Read the model definition and answer for the solid it produces. Units are mm, in the model's axes. Face numbers are marked on the shaded views. A direction names the side the tool comes from. Give positions to 0.01 mm unless a question says otherwise; leave off trailing zeros. Write each loop counter-clockwise with the first axis right and the second up, starting at its lowest first coordinate (ties: lowest second). Pieces come first, ordered by that corner, then holes. Notation, with made-up numbers: M -8.5,-28.75 L 5.5,-28.75 A17 ccw 5.5,-11.75 Z; hole C 25.5,-8 d8. An arc over 180 degrees is marked long. Put each result on its own line as item: value.
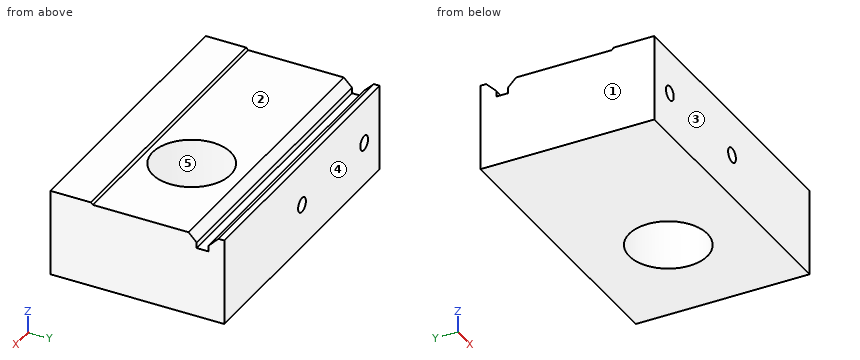
from build123d import *

# Parameters (mm, degrees)
SKETCH1_W                   = 100
SKETCH1_H                   = 60
BOSS_EXTRUDE1_DEPTH         = 30
CUT_EXTRUDE1_DEPTH          = 110
SKETCH_1_R                  = 2.5
CUT_EXTRUDE_1_DEPTH         = 10
PATTERN_LINEAR_1_COUNT      = 2
PATTERN_LINEAR_1_PITCH      = 40
PATTERN_LINEAR_1_COUNT_DIR2 = 2
PATTERN_LINEAR_1_PITCH_DIR2 = 50
SKETCH_2_R                  = 13.5
CUT_EXTRUDE_2_DEPTH         = 100


with BuildPart() as part:
    # Sketch1 → Boss-Extrude1 (new body)
    with BuildSketch(Plane.XY):
        with Locations((2.079207921, -0.485148515)):
            Rectangle(SKETCH1_W, SKETCH1_H)
    extrude(amount=BOSS_EXTRUDE1_DEPTH)

    # Sketch3 → Cut-Extrude1 (cut)
    with BuildSketch(Plane.ZY.offset(47.920792079)):
        Polygon((30, -30.485148515), (30, -16.485148515), (29.292893219, -15.778041734), (29.292893219, 17.150890454), (26.464466094, 19.979317579), (24.464466094, 19.979317579), (24.464466094, 23.979317579), (26.464466094, 23.979317579), (30, 27.514851485), (30, 29.514851485), (35.630972976, 28.601630178), (37.149112702, -26.247837132), align=None)
    extrude(amount=-CUT_EXTRUDE1_DEPTH, mode=Mode.SUBTRACT)

    # Эскиз1 → Вырез-Вытянуть1 (cut)
    with BuildSketch(Plane(origin=(0, 29.514851485, 0), x_dir=(1, 0, 0), z_dir=(0, 1, 0))):
        with Locations((2.079207921, -15)):
            Circle(SKETCH_1_R)
    cut_extrude_1 = extrude(amount=-CUT_EXTRUDE_1_DEPTH, mode=Mode.SUBTRACT)

    # Линейный массив1: Cut-Extrude 1 2 × 2
    with Locations(*[(-i * PATTERN_LINEAR_1_PITCH, -j * PATTERN_LINEAR_1_PITCH_DIR2, 0) for i in range(PATTERN_LINEAR_1_COUNT) for j in range(PATTERN_LINEAR_1_COUNT_DIR2) if (i, j) != (0, 0)]):
        add(cut_extrude_1, mode=Mode.SUBTRACT)

    # Эскиз2 → Вырез-Вытянуть2 (cut)
    with BuildSketch(Plane(origin=(0, 0, 0), x_dir=(-1, 0, 0), z_dir=(0, 0, -1))):
        with Locations((-17.079207921, -0.485148515)):
            Circle(SKETCH_2_R)
    extrude(amount=-CUT_EXTRUDE_2_DEPTH, mode=Mode.SUBTRACT)


solid = part.part
(1) Section D-D on x = 19 is taken. Determine the outline of the cut face in (y, z), and give its area (3 significant figures).
Result:
outline: M -30.49,0 L -13.85,0 L -13.85,29.29 L -15.78,29.29 L -16.49,30 L -30.49,30 Z; M 12.88,0 L 29.51,0 L 29.51,30 L 27.51,30 L 23.98,26.46 L 23.98,24.46 L 19.98,24.46 L 19.98,26.46 L 17.15,29.29 L 12.88,29.29 Z
area: 959 mm²
(2) Section C-C on z = 15 is taken. Determine the outline of the cut face in (x, y), and give its area (3 significant figures).
Result:
outline: M -47.92,-30.49 L -40.42,-30.49 L -40.42,-20.49 L -35.42,-20.49 L -35.42,-30.49 L -0.42,-30.49 L -0.42,-20.49 L 4.58,-20.49 L 4.58,-30.49 L 52.08,-30.49 L 52.08,29.51 L 4.58,29.51 L 4.58,19.51 L -0.42,19.51 L -0.42,29.51 L -35.42,29.51 L -35.42,19.51 L -40.42,19.51 L -40.42,29.51 L -47.92,29.51 Z; hole C 17.08,-0.49 d27
area: 5,230 mm²
(3) Section A-A on y = 21 is taken. Determine the outline of the cut face in (x, z).
Result:
outline: M -47.92,0 L 52.08,0 L 52.08,24.46 L -47.92,24.46 Z; hole C -37.92,15 d5; hole C 2.08,15 d5
(4) Given pin 1 Ø5.5 at (x, z) = (-38, 16) entering from -Y; pin 2 Ø4 at (x, z) = (-37.92, 15) entering from -Y; pin 3 Ø3 at (x, y) = (-15.5, 22) entering from +Z; pin 4 Ø2.5 at (x, z) = (1.5, 16) entering from +Y, each flat-ended and moving along its own axis, determine where each tip first touches the part or whether it passes through.
Result:
pin 1: stops at y = -30.49
pin 2: stops at y = -20.49
pin 3: stops at z = 24.46
pin 4: stops at y = 19.51
(5) Straight lines are drawn through the part: line 1 along X through (y, z) = (-27.5, 15); line 2 along Y through (x, z) = (-28.5, 26.25); line 3 along Z through (x, y) = (-44, 21.5). For each, find the intervals that lie inside material, in ascending order. Write a range as from..to.
Result:
line 1: x = -47.92..-40.42, -35.42..-0.42, 4.58..52.08
line 2: y = -30.49..19.98, 23.98..29.51
line 3: z = 0..24.46
(6) Section B-B on x = -2.5 is taken. Determine the outline of the cut face in (y, z).
Result:
outline: M -30.49,0 L 29.51,0 L 29.51,30 L 27.51,30 L 23.98,26.46 L 23.98,24.46 L 19.98,24.46 L 19.98,26.46 L 17.15,29.29 L -15.78,29.29 L -16.49,30 L -30.49,30 Z
(7) For a pull along Y with two mould halves and no side action, classify the marked faces 3, 4 and 5 as +Y half, -Y half, draft (parallel to the pull), parting line (faces both ways), or undercut.
Result:
face 3: -Y half
face 4: +Y half
face 5: undercut
(8) Which of the six approach directions +Z, -Z, +X, -X, +Y, -Y give full straight-line access (tool end or side, diameter ignored) to the marked faces 1 and 2?
Result:
face 1: +Z, -Z, -X, +Y, -Y
face 2: +Z, +X, -X
